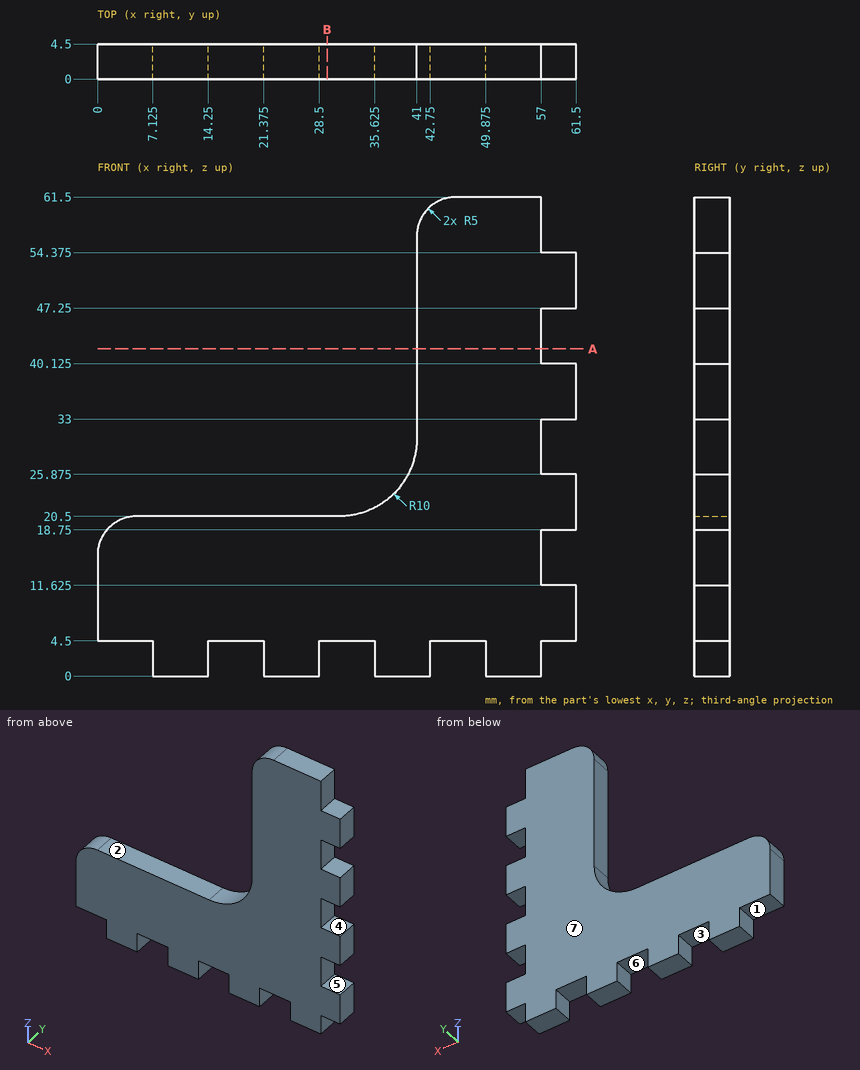
Geometry check sheet. Reference: drawing and pictorial views, mm from the part's lowest x, y, z. A direction names the side the tool comes from. Give positions to 0.01 mm unless a question says otherwise; leave off trailing zeros. Write each loop counter-clockwise with the first axis right and the second up, starting at its lowest first coordinate (ties: lowest second). Pieces come first, ordered by that corner, then holes. Notation, with made-up numbers: M -30.5,80 L 17.5,80 A12 cw 17.5,94 Z; hole C 89,43.25 d5. An arc over 180 degrees is marked long. Use CSV: the item, a comma, the result in double quotes.
1) Cross-section at B-B (x = 29.5). Enter the section's corners in (y, z), plus the area to 3 significant figures.
Final values:
outline,"M 0,4.5 L 4.5,4.5 L 4.5,20.5 L 0,20.5 Z"
area,"72.0 mm²"
2) Go/stop test with flat-tipped pins: pin 1 Ø1.3 at (x, y) = (60.5, 3) entering from +Z (3 decimals); pin 2 Ø2 at (y, z) = (3, 2.5) entering from -X (3 decimals); pin 3 Ø1.3 at (x, y) = (59.5, 3) entering from -Z; pin 4 Ø6 at (x, z) = (37, 51.5) entering from -Y. Record where each tip stops, or that it passes through.
Final values:
pin 1,"z = 54.375"
pin 2,"x = 7.125"
pin 3,"z = 4.5"
pin 4,"through"
3) Release check for a two-part mould opening along Z. For the marked faces 5, 6 and 7 record: released by +Z, released by -Z, zero draft, split by the parting line, or undercut.
Final values:
face 5,"undercut"
face 6,"released by -Z"
face 7,"zero draft"
4) Material ranges on line 1 along X through (y, z) = (4.1, 3) (3 decimals); line 2 along Z through (x, y) = (23, 3.2); line 3 along X through (y, z) = (4.05, 12.5), recorded low to high.
Final values:
line 1,"7.125 to 14.25, 21.375 to 28.5, 35.625 to 42.75, 49.875 to 57"
line 2,"0 to 20.5"
line 3,"0 to 57"
5) Cross-section at A-A (z = 42). Enter the section's corners in (x, y).
Final values:
outline,"M 41,0 L 57,0 L 57,4.5 L 41,4.5 Z"
6) Access from +Z, -Z, +X, -X, +Y, -Y to the whole of each face (thin tool, end or side, straight path). Record for the marked faces 1, 2, 3 and 4.
Final values:
face 1,"-Z, -X, +Y, -Y"
face 2,"+Z, -X, +Y, -Y"
face 3,"-Z, +Y, -Y"
face 4,"+X, +Y, -Y"
